Part print with two shaded views. Sizes in mm from the minimum x, y, z corner. A direction names the side the tool comes from. Round coordinates to 2 decimals unless told otherwise and drop trailing zeros. Loops run counter-clockwise (first coordinate to the right, second up) from the corner with the lowest first, then second, coordinate; pieces in that order, holes last.
(1) Cut at D-D on y = 14.5. List the corners of the cut face in (x, z).
(2) Flat gauge pins, fed straight in: pin 1 (8 mm diameter, centred on x = 11.5, y = 12.5, fed in from +Z); pin 2 (2.5 mm diameter, centred on x = 10.75, y = 8.08, fed in from +Z); pin 3 (1.5 mm diameter, centred on x = 28, z = 17.5, fed in from +Y). Where does each tip first touch, or does it go through?
(3) Tool access for the marked faces 1 and 2: list every direction of +Z, -Z, +X, -X, +Y, -Y with a clear straight run to the whole face (end or side of a thin tool).
(4) Cut at C-C on x = 35. List the corners of the cut face in (y, z), then the cut area to 3 significant figures.
(5) Cut at B-B on y = 21.5. List the corners of the cut face in (x, z).
(6) Probe probe 1 along Z at (x, y) = (7, 1.5); probe 2 along Y at (x, z) = (10.75, 1.45); probe 3 along X at (y, z) = (6.75, 2.5). List the from-to ranges inside material, lowest first.
(7) Cut at A-A on z = 9.75. List the corners of the cut face in (x, y).
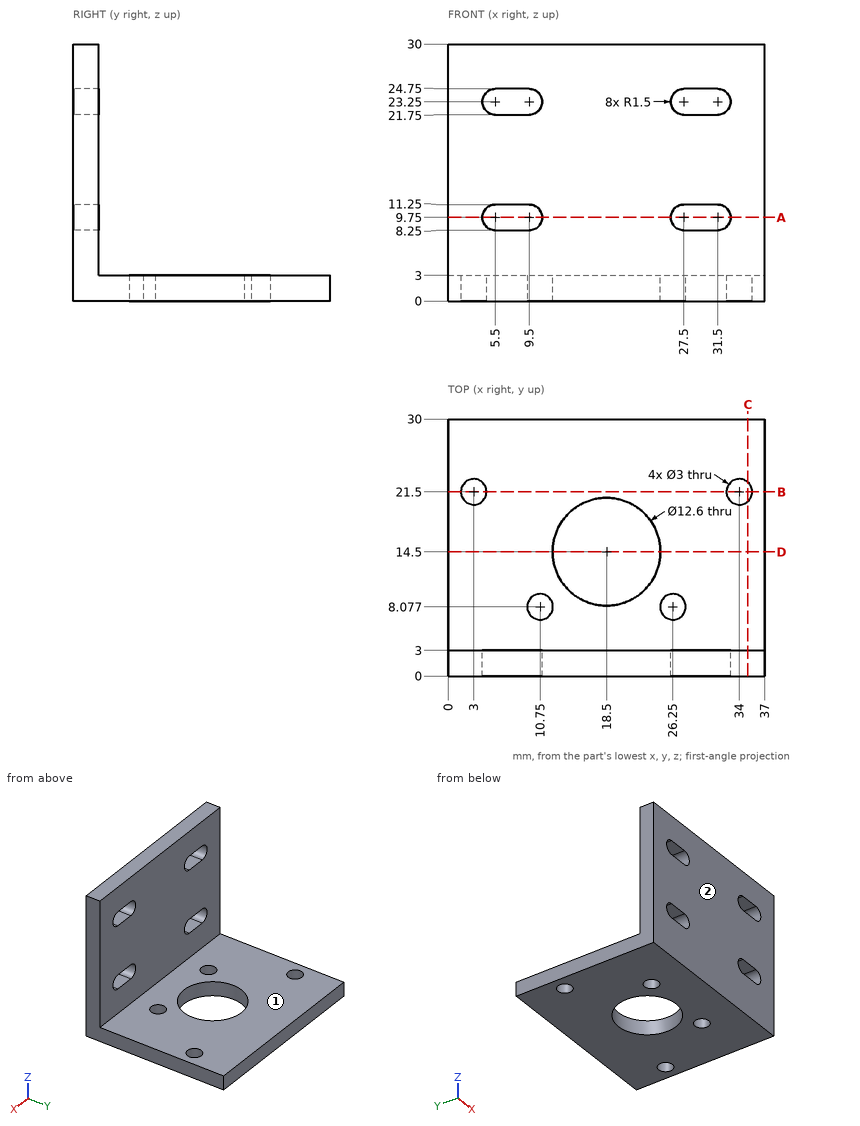
Final values:
1. outline: (0, 0) - (12.2, 0) - (12.2, 3) - (0, 3) - close; (24.8, 0) - (37, 0) - (37, 3) - (24.8, 3) - close
2. pin 1: stops at z = 3
2. pin 2: passes through
2. pin 3: stops at y = 3
3. face 1: +Z, +X, -X, +Y
3. face 2: +Z, -Z, +X, -X, -Y
4. outline: (0, 0) - (20.38, 0) - (20.38, 3) - (3, 3) - (3, 30) - (0, 30) - close; (22.62, 0) - (30, 0) - (30, 3) - (22.62, 3) - close
4. area: 164 mm2
5. outline: (0, 0) - (1.5, 0) - (1.5, 3) - (0, 3) - close; (4.5, 0) - (32.5, 0) - (32.5, 3) - (4.5, 3) - close; (35.5, 0) - (37, 0) - (37, 3) - (35.5, 3) - close
6. probe 1: z = 0 to 8.25, 11.25 to 21.75, 24.75 to 30
6. probe 2: y = 0 to 6.58, 9.58 to 30
6. probe 3: x = 0 to 10.05, 11.45 to 25.55, 26.95 to 37
7. outline: (0, 0) - (4, 0) - (4, 3) - (0, 3) - close; (11, 0) - (26, 0) - (26, 3) - (11, 3) - close; (33, 0) - (37, 0) - (37, 3) - (33, 3) - close
